CAD build for the part. Positions are in the model's coordinates, mm. A direction names the side the tool comes from. Round coordinates to 2 decimals unless told otherwise and drop trailing zeros. Loops run counter-clockwise (first coordinate to the right, second up) from the corner with the lowest first, then second, coordinate; pieces in that order, holes last. Notation, with made-up numbers: (48.5, -36.5) - (92.5, -36.5) arc R26 ccw to (92.5, -3.5) - close; hole circle Ø10 at (68.5, -1.75). An arc over 180 degrees is marked (long way). One line per question, with ' | ' between items.
```python
from build123d import *

# Parameters (mm, degrees)
SKETCH1_W                = 40
SKETCH1_H                = 240
BOSS_EXTRUDE1_DEPTH      = 6
SKETCH3_W                = 73.413063841
SKETCH3_H                = 6
BOSS_EXTRUDE2_DEPTH      = 10
BOSS_EXTRUDE2_DEPTH_BACK = 50
SKETCH4_W                = 28
SKETCH4_H                = 14
BOSS_EXTRUDE3_DEPTH      = 8
SKETCH5_W                = 14
SKETCH5_H                = 2
BOSS_EXTRUDE4_DEPTH      = 2
BOSS_EXTRUDE4_DEPTH_BACK = 30
CUT_EXTRUDE1_DEPTH       = 10


with BuildPart() as part:
    # Sketch1 → Boss-Extrude1 (new body)
    with BuildSketch(Plane(origin=(0, 0, 0), x_dir=(1, 0, 0), z_dir=(0, 1, 0))):
        Rectangle(SKETCH1_W, SKETCH1_H)
    extrude(amount=BOSS_EXTRUDE1_DEPTH)

    # Sketch3 → Boss-Extrude2 (add, two sides)
    with BuildSketch(Plane(origin=(20, 0, 0), x_dir=(0, 0, -1), z_dir=(1, 0, 0))) as boss_extrude2_sk:
        with Locations((-83.29346808, 3)):
            Rectangle(SKETCH3_W, SKETCH3_H)
    extrude(amount=BOSS_EXTRUDE2_DEPTH)
    extrude(boss_extrude2_sk.sketch, amount=-BOSS_EXTRUDE2_DEPTH_BACK)

    # Sketch4 → Boss-Extrude3 (add)
    with BuildSketch(Plane.XZ):
        with Locations((0, -103)):
            Rectangle(SKETCH4_W, SKETCH4_H)
    extrude(amount=BOSS_EXTRUDE3_DEPTH)

    # Sketch5 → Boss-Extrude4 (add, two sides)
    with BuildSketch(Plane(origin=(14, 0, 0), x_dir=(0, 0, -1), z_dir=(1, 0, 0))) as boss_extrude4_sk:
        with Locations((103, -7)):
            Rectangle(SKETCH5_W, SKETCH5_H)
    extrude(amount=BOSS_EXTRUDE4_DEPTH)
    extrude(boss_extrude4_sk.sketch, amount=-BOSS_EXTRUDE4_DEPTH_BACK)

    # Sketch2 → Cut-Extrude1 (cut)
    with BuildSketch(Plane.XZ):
        with BuildLine():
            Line((-2.05, 99.374369573), (2.05, 99.374369573))
            ThreePointArc((2.05, 99.374369573), (2.540177159, 100.874369573), (2.05, 102.374369573))
            Line((2.05, 102.374369573), (-2.05, 102.374369573))
            ThreePointArc((-2.05, 102.374369573), (-2.540177159, 100.874369573), (-2.05, 99.374369573))
        make_face()
        with BuildLine():
            ThreePointArc((-21.42, 100.874369573), (-20.718261003, 95.436533515), (-18.659023249, 90.354994526))
            ThreePointArc((-18.659023249, 90.354994526), (-19.457027975, 87.494367242), (-22.317655259, 88.292371968))
            ThreePointArc((-22.317655259, 88.292371968), (-24.780665122, 94.37029115), (-25.62, 100.874369573))
            ThreePointArc((-25.62, 100.874369573), (-24.814500332, 107.248141867), (-22.44865158, 113.221127942))
            ThreePointArc((-22.44865158, 113.221127942), (-19.596568798, 114.049151976), (-18.768544764, 111.197069193))
            ThreePointArc((-18.768544764, 111.197069193), (-20.746549458, 106.203261163), (-21.42, 100.874369573))
        make_face()
        with BuildLine():
            ThreePointArc((25.62, 100.874369573), (24.780665122, 94.37029115), (22.317655259, 88.292371968))
            ThreePointArc((22.317655259, 88.292371968), (19.457027975, 87.494367242), (18.659023249, 90.354994526))
            ThreePointArc((18.659023249, 90.354994526), (20.718261003, 95.436533515), (21.42, 100.874369573))
            ThreePointArc((21.42, 100.874369573), (20.746549458, 106.203261163), (18.768544764, 111.197069193))
            ThreePointArc((18.768544764, 111.197069193), (19.596568798, 114.049151976), (22.44865158, 113.221127942))
            ThreePointArc((22.44865158, 113.221127942), (24.814500332, 107.248141867), (25.62, 100.874369573))
        make_face()
    extrude(amount=-CUT_EXTRUDE1_DEPTH, mode=Mode.SUBTRACT)


solid = part.part
```
(1) Two-plate mould, pull along X, no slides. Class faces 1 (the face through (14, -3, -103)), 2 (the face through (0, 3, 102.374)), 3 (the face through (0, 3, 120)): released by +X, released by -X, zero draft, split by the parting line, or undercut.
Results found:
face 1: released by +X | face 2: undercut | face 3: zero draft
(2) Tool access for faces 4 (the face through (0, 3, 99.374)), 5 (the face through (0, -4, -96)), 6 (the face through (-14, -3, -103)), 7 (the face through (-25, 3, 46.587)), 8 (the face through (25, 3, 46.587)): list every direction of +Z, -Z, +X, -X, +Y, -Y with a clear straight run to the whole face (end or side of a thin tool).
Results found:
face 4: +Y, -Y | face 5: +Z, +X, -X, -Y | face 6: +Z, -Z, -X | face 7: -Z, -X, +Y, -Y | face 8: -Z, +X, +Y, -Y
(3) Cut at C-C, the plane z = -14.5. Write the cut outline in (x, y), then the cut area to 3 significant figures.
Results found:
outline: (-20, 0) - (20, 0) - (20, 6) - (-20, 6) - close | area: 240 mm²
(4) Cut at A-A, the plane y = 2.5. Write the cut outline in (x, z) (3 decimals).
Results found:
outline: (-30, 46.587) - (-20, 46.587) - (-20, -120) - (20, -120) - (20, 46.587) - (30, 46.587) - (30, 120) - (-30, 120) - close; hole (-22.449, 113.221) arc R25.62 ccw to (-22.318, 88.292) arc R2.1 ccw to (-18.659, 90.355) arc R21.42 cw to (-18.769, 111.197) arc R2.1 ccw to start; hole (-2.05, 99.374) - (2.05, 99.374) arc R2.54 ccw to (2.05, 102.374) - (-2.05, 102.374) arc R2.54 ccw to start; hole (18.659, 90.355) arc R2.1 ccw to (22.318, 88.292) arc R25.62 ccw to (22.449, 113.221) arc R2.1 ccw to (18.769, 111.197) arc R21.42 cw to start
(5) Probe L1, parallel to Z at x = 11, y = -2.5; L2, parallel to Y at x = -3, z = -26.5; L3, parallel to X at y = 5.25, z = 38. List the from-to ranges inside material, lowest first.
Results found:
L1: z = -110 to -96 | L2: y = 0 to 6 | L3: x = -20 to 20
(6) Cut at D-D, the plane z = 83.5. Write the cut outline in (x, y).
Results found:
outline: (-30, 0) - (30, 0) - (30, 6) - (-30, 6) - close
(7) Cut at B-B, the plane x = 7. Write the cut outline in (y, z), then the cut area to 3 significant figures.
Results found:
outline: (-8, -110) - (0, -110) - (0, -120) - (6, -120) - (6, 120) - (0, 120) - (0, -96) - (-8, -96) - close | area: 1,550 mm²
(8) Drop flat-ended pins along their axis: P1, Ø4, axis at y = 4.5, z = -20.5, coming from the -X side; P2, Ø6.5, axis at x = 2, y = -5.5, coming from the +Z side; P3, Ø5, axis at y = 1.5, z = -4, coming from the +X side. Give the stop position or say it passes through.
Results found:
P1: stops at x = -20 | P2: stops at z = -96 | P3: stops at x = 20
